Could you check a few things on this model? Use its own coordinates, in mm. Give positions to 0.01 mm unless a question says otherwise; leave off trailing zeros. Order: outer loops, then holes, each group sorted by start corner. A loop starts at its lowest first (then second) coordinate and runs counter-clockwise, first axis right, second up.
from build123d import *

# Parameters (mm, degrees)
SKETCH1_W               = 3.556
SKETCH1_H               = 95.25
BOSS_EXTRUDE1_DEPTH     = 1.399999994
BOSS_EXTRUDE2_START     = -2.799999988
BOSS_EXTRUDE2_DEPTH     = 2.799999988
CUT_EXTRUDE1_DEPTH      = 96.57729743
CUT_EXTRUDE1_DEPTH_BACK = 96.57729743


# Read off the part's stored shape, not the designer's step: Boss-Extrude2
with BuildPart() as part:
    # Sketch1 → Boss-Extrude1 (new, symmetric)
    with BuildSketch(Plane(origin=(0, 0, 0), x_dir=(1, 0, 0), z_dir=(0, 1, 0))):
        Rectangle(SKETCH1_W, SKETCH1_H)
    extrude(amount=BOSS_EXTRUDE1_DEPTH, both=True)

    # Boss-Extrude2 outline → Boss-Extrude2 (add)
    with BuildSketch(Plane(origin=(0, 1.399999994, 0), x_dir=(1, 0, 0), z_dir=(0, 1, 0)).offset(BOSS_EXTRUDE2_START)):
        Polygon((-1.778, 47.625), (-5.746, 47.625), (-7.778, 47.117), (-7.778, 41.783), (-5.746, 41.275), (-1.778, 41.275), align=None)
        Polygon((3.762000096, 34.925), (1.778, 34.925), (1.778, 28.575), (3.526821698, 28.575), (4.778000096, 29.200589199), (4.778000096, 34.417), align=None)
        Polygon((-1.778, 15.875), (-1.778, 22.225), (-5.746, 22.225), (-7.778, 21.717), (-7.778, 16.383), (-5.746, 15.875), align=None)
        Polygon((3.762000096, -15.875), (1.778, -15.875), (1.778, -22.225), (3.526821698, -22.225), (4.778000096, -21.599410801), (4.778000096, -16.383), align=None)
        Polygon((-1.778, -22.225), (-1.778, -15.875), (-5.746, -15.875), (-7.778, -16.383), (-7.778, -21.717), (-5.746, -22.225), align=None)
        Polygon((-1.778, -47.625), (-1.778, -41.275), (-5.746, -41.275), (-7.778, -41.783), (-7.778, -47.117), (-5.746, -47.625), align=None)
    extrude(amount=BOSS_EXTRUDE2_DEPTH)

    # Sketch3 → Cut-Extrude1 (cut, two sides: drawn at the far end of the back side and taken through both)
    with BuildSketch(Plane.XY.offset(47.625).offset(-CUT_EXTRUDE1_DEPTH_BACK)):
        Polygon((-7.778, 0.891999994), (-6.254, 1.399999994), (-7.778, 1.399999994), align=None)
        Polygon((4.778000096, 1.145999994), (4.778000096, 1.399999994), (3.762000096, 1.399999994), align=None)
    extrude(amount=CUT_EXTRUDE1_DEPTH + CUT_EXTRUDE1_DEPTH_BACK, mode=Mode.SUBTRACT)


solid = part.part
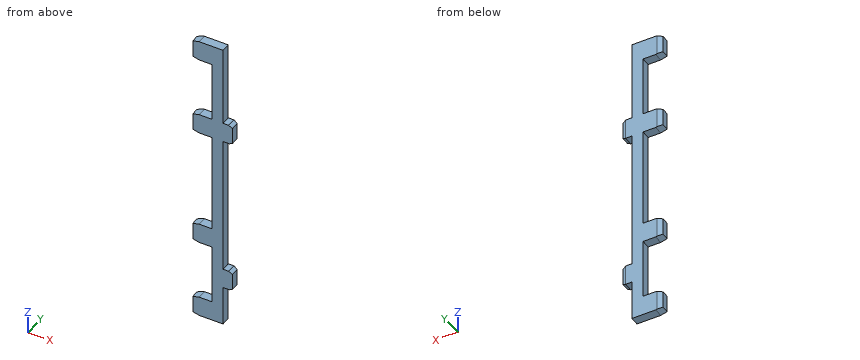
Item 1: For pin 1 (0.6 mm diameter, centred on x = 3, y = 0, fed in from -Z) (3 decimals); pin 2 (0.8 mm diameter, centred on y = -0.5, z = 28, fed in from -X); pin 3 (0.9 mm diameter, centred on x = 2.5, y = 0, fed in from +Z) (3 decimals), each with a flat end and sliding along its axis, tell me the tip position at first contact or that it passes through.
Findings:
pin 1: stops at z = -34.925
pin 2: stops at x = -1.78
pin 3: stops at z = 22.225
Item 2: Imagine slicing it at A-A on x = -3.5. List the corners of the cut face in (y, z) for me (3 decimals).
Findings:
outline: (-1.4, -47.625) - (1.4, -47.625) - (1.4, -41.275) - (-1.4, -41.275) - close; (-1.4, -22.225) - (1.4, -22.225) - (1.4, -15.875) - (-1.4, -15.875) - close; (-1.4, 15.875) - (1.4, 15.875) - (1.4, 22.225) - (-1.4, 22.225) - close; (-1.4, 41.275) - (1.4, 41.275) - (1.4, 47.625) - (-1.4, 47.625) - close
Item 3: Imagine slicing it at C-C on z = 31. List the corners of the cut face in (x, y) for me.
Findings:
outline: (-1.78, -1.4) - (1.78, -1.4) - (1.78, 1.4) - (-1.78, 1.4) - close
Item 4: Please list where these lines run through material, in increasing order: line 1 along Z through (x, y) = (-4.5, 0.65) (3 decimals); line 2 along X through (y, z) = (-0.8, 8.5); line 3 along Z through (x, y) = (3.75, -0.1) (3 decimals).
Findings:
line 1: z = -47.625 to -41.275, -22.225 to -15.875, 15.875 to 22.225, 41.275 to 47.625
line 2: x = -1.78 to 1.78
line 3: z = -34.925 to -28.687, 15.875 to 22.113
Item 5: Imagine slicing it at B-B on z = -32. List the corners of the cut face in (x, y) for me, then the cut area to 3 significant figures.
Findings:
outline: (-1.78, -1.4) - (4.78, -1.4) - (4.78, 1.15) - (3.76, 1.4) - (-1.78, 1.4) - close
area: 18.2 mm2
